Here's how the part is built. I have some questions about the finished solid (model axes, mm). Face numbers are marked on the shaded views. A direction names the side the tool comes from. Give positions to 0.01 mm unless a question says otherwise; leave off trailing zeros. Loops run counter-clockwise (first coordinate to the right, second up) from the corner with the lowest first, then second, coordinate; pieces in that order, holes last. Notation, with made-up numbers: M -39,-12.5 L 20,-12.5 A36 cw 20,26.5 Z; hole C -15,-31.75 d1. An arc over 180 degrees is marked long. Answer as CSV lines item,"result". Start each with the question number.
Item 1: For the marked faces 5, 6 and 7, which set-ups out of +Z, -Z, +X, -X, +Y, -Y let a thin tool reach every point of the face, with its end or its side?
Item 2: I want a section at D-D on x = -10.5. List the corners of the cut face in (y, z) for me, plus the area to 3 significant figures.
Item 3: If I drill on line 1 along Z through (x, y) = (7, -9.1); line 2 along X through (y, z) = (-3.5, 10.75); line 3 along X through (y, z) = (-10, 11), over which ranges is the centre line in solid material (lowest first)? Write a range as from..to.
Item 4: I want a section at A-A on z = 7.5. List the corners of the cut face in (x, y) for me, plus the area to 3 significant figures.
Item 5: If we mould it in two halves opening along Y, with no side actions, what happens to the marked faces 1, 2, 3 and 4? For each: released by +Y, released by -Y, zero draft, split by the parting line, or undercut.
Item 6: Will these pins go through, and if not, where does the flat tip stop? P1, Ø6, axis at x = 7, z = 7.5, coming from the -Y side; P2, Ø9, axis at x = -7, z = 7.5, coming from the +Y side.
Item 7: I want a section at B-B on y = -9. List the corners of the cut face in (x, z) for me.
Item 8: I want a section at C-C on z = 13. List the corners of the cut face in (x, y) for me, plus the area to 3 significant figures.
from build123d import *

# Parameters (mm, degrees)
CROQUIS2_W              = 30
CROQUIS2_H              = 17.375045376
SALIENTE_EXTRUIR1_DEPTH = 2
CROQUIS3_R              = 4.25
SALIENTE_EXTRUIR2_DEPTH = 13
CROQUIS4_R              = 5
CORTAR_EXTRUIR1_DEPTH   = 4.6


with BuildPart() as part:
    # Croquis2 → Saliente-Extruir1 (new body)
    with BuildSketch(Plane.XY):
        with Locations((0, -3.687522688)):
            Rectangle(CROQUIS2_W, CROQUIS2_H)
    extrude(amount=SALIENTE_EXTRUIR1_DEPTH)

    # Croquis3 → Saliente-Extruir2 (add)
    with BuildSketch(Plane.XY.offset(2)):
        Circle(CROQUIS3_R)
        with BuildLine():
            Line((-15, 5), (-14.271293534, 5))
            ThreePointArc((-14.271293534, 5), (-9.727126272, 3.291298824), (-7.434621256, -0.98813298))
            ThreePointArc((-7.434621256, -0.98813298), (0, -7.5), (7.434621256, -0.98813298))
            ThreePointArc((7.434621256, -0.98813298), (9.727126272, 3.291298824), (14.271293534, 5))
            Line((14.271293534, 5), (15, 5))
            Line((15, 5), (15, -12.375045376))
            Line((15, -12.375045376), (-15, -12.375045376))
            Line((-15, -12.375045376), (-15, 5))
        make_face()
    extrude(amount=SALIENTE_EXTRUIR2_DEPTH)

    # Croquis4 → Cortar-Extruir1 (cut)
    with BuildSketch(Plane.XZ.offset(12.375045376)):
        with Locations((-7, 7.5)):
            Circle(CROQUIS4_R)
        with Locations((7, 7.5)):
            Circle(CROQUIS4_R)
    extrude(amount=-CORTAR_EXTRUIR1_DEPTH, mode=Mode.SUBTRACT)


solid = part.part
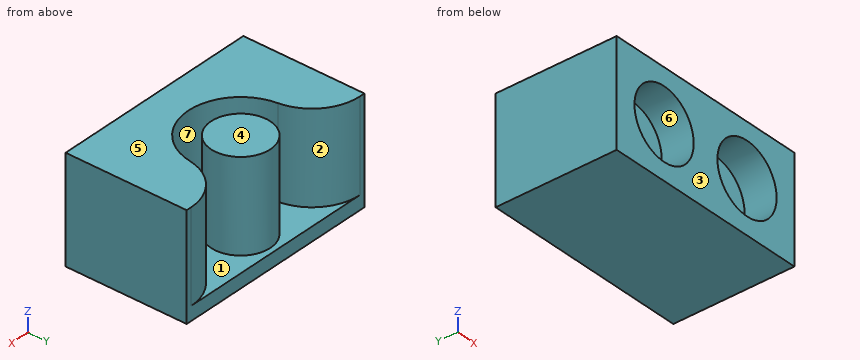
Result:
1,face 5,"+Z, +X, -X, +Y, -Y"
1,face 6,"-Y"
1,face 7,"+Z"
2,outline,"M -12.38,0 L 5,0 L 5,2 L 3.88,2 L 3.88,15 L -12.38,15 L -12.38,11.07 L -7.78,11.07 L -7.78,3.93 L -12.38,3.93 Z"
2,area,"213 mm^2"
3,line 1,"0..2.5, 12.5..15"
3,line 2,"-15..-6.63, -2.41..2.41, 6.63..15"
3,line 3,"-15..-10.57, -3.43..3.43, 10.57..15"
4,outline,"M -15,-12.38 L -12,-12.38 L -12,-7.78 L -2,-7.78 L -2,-12.38 L 2,-12.38 L 2,-7.78 L 12,-7.78 L 12,-12.38 L 15,-12.38 L 15,5 L 14.27,5 A6.9 ccw 7.43,-0.99 A7.5 cw -7.43,-0.99 A6.9 ccw -14.27,5 L -15,5 Z; C 0,0 d8.5"
4,area,"304 mm^2"
5,face 1,"undercut"
5,face 2,"released by +Y"
5,face 3,"released by -Y"
5,face 4,"zero draft"
6,P1,"y = -7.78"
6,P2,"y = 4.42"
7,outline,"M -15,0 L 15,0 L 15,15 L -15,15 Z; hole C -7,7.5 d10; hole C 7,7.5 d10"
8,outline,"M -15,-12.38 L 15,-12.38 L 15,5 L 14.27,5 A6.9 ccw 7.43,-0.99 A7.5 cw -7.43,-0.99 A6.9 ccw -14.27,5 L -15,5 Z; C 0,0 d8.5"
8,area,"396 mm^2"
